The listing builds one solid part. Answer for the finished solid, in the listing's coordinates (mm). Face numbers are marked on the shaded views. A direction names the side the tool comes from. Coordinates: 2 decimals unless noted, no trailing zeros. Write each loop counter-clockwise with the first axis right and the second up, starting at its lowest first coordinate (ties: lowest second). Pieces come first, ordered by that corner, then holes.
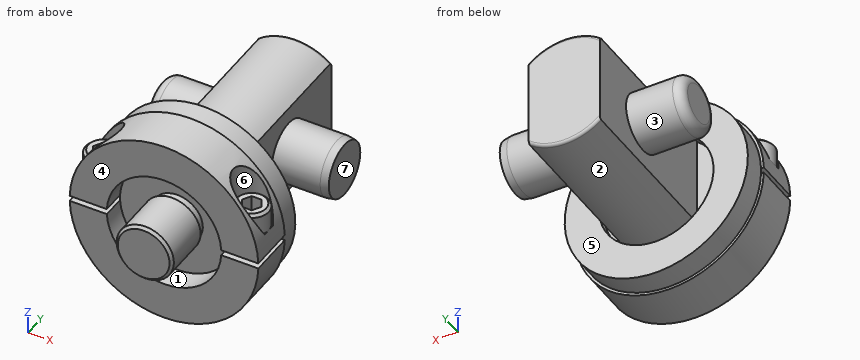
from build123d import *

# Parameters (mm, degrees)
FILLET1_R                  = 0.7874
SKETCH2_W                  = 6.0198
SKETCH2_H                  = 46.736
CUT_EXTRUDE1_DEPTH         = 16.875
CUT_EXTRUDE1_DEPTH_BACK    = 16.875
SKETCH3_R                  = 7.9375
SKETCH3_R_2                = 7.0866
CUT_EXTRUDE2_DEPTH         = 2.54
CHAMFER1_SIZE              = 0.762
SKETCH4_R                  = 7.94004
EXTRUDE1_DEPTH             = 25.4
CHAMFER2_SIZE              = 0.381
CHAMFER2_SIZE2             = 2.160758373
FILLET2_R                  = 2.6416
EXTRUDE2_DEPTH             = 6.35
EXTRUDE2_DEPTH_BACK        = 6.35
CUT_EXTRUDE3_START         = 5.588
SKETCH6_R                  = 5.1562
CUT_EXTRUDE3_DEPTH         = 20.812
SKETCH7_R                  = 4.7625
EXTRUDE3_DEPTH             = 6.35
CHAMFER3_SIZE              = 0.762
CUT_EXTRUDE4_DEPTH         = 4.7625
EXTRUDE4_REACH             = 28.162
SKETCH10_R                 = 3.175
EXTRUDE4_DIRECTION_2_REACH = 28.162
SKETCH11_R                 = 25.4
SKETCH11_R_2               = 15.875
EXTRUDE5_DEPTH             = 6.35


with BuildPart() as part:
    # Sketch1 → Revolve1 (revolve)
    with BuildSketch(Plane(origin=(0, 0, 0), x_dir=(0, 0, -1), z_dir=(1, 0, 0))):
        Polygon((0, 56.896), (15.875, 56.896), (15.875, 0), (7.9375, 0), (7.9375, -16.129), (0, -16.129), align=None)
    revolve(axis=Axis((0, -15.35938, 0), (0, 1, 0)))

    # Fillet1
    fillet1_edges = [part.edges().sort_by_distance(p)[0] for p in [
        (0, 56.896, 15.875),
    ]]
    fillet(fillet1_edges, radius=FILLET1_R)

    # Sketch2 → Cut-Extrude1 (cut, two sides)
    with BuildSketch(Plane.XY) as cut_extrude1_sk:
        with Locations((12.8651, 33.528)):
            Rectangle(SKETCH2_W, SKETCH2_H)
        with Locations((-12.8651, 33.528)):
            Rectangle(SKETCH2_W, SKETCH2_H)
    extrude(amount=CUT_EXTRUDE1_DEPTH, mode=Mode.SUBTRACT)
    extrude(cut_extrude1_sk.sketch, amount=-CUT_EXTRUDE1_DEPTH_BACK, mode=Mode.SUBTRACT)

    # Sketch3 → Cut-Extrude2 (cut)
    with BuildSketch(Plane.XZ):
        with Locations(Location((0, 0, 0), (0, 0, 270))):  # turned: the seam where the file's is
            Circle(SKETCH3_R)
        with Locations(Location((0, 0, 0), (0, 0, 270))):  # turned: the seam where the file's is
            Circle(SKETCH3_R_2, mode=Mode.SUBTRACT)
    extrude(amount=CUT_EXTRUDE2_DEPTH, mode=Mode.SUBTRACT)

    # Chamfer1
    chamfer1_edges = [part.edges().sort_by_distance(p)[0] for p in [
        (0, -16.129, 7.9375),
    ]]
    chamfer(chamfer1_edges, length=CHAMFER1_SIZE)

    # Sketch4 → Extrude1 (add, symmetric)
    with BuildSketch(Plane(origin=(0, 0, 0), x_dir=(0, 0, -1), z_dir=(1, 0, 0))):
        with Locations(Location((0, 36.322, 0), (0, 0, 90))):  # turned: the seam where the file's is
            Circle(SKETCH4_R)
    extrude(amount=EXTRUDE1_DEPTH, both=True)

    # Chamfer2
    chamfer2_edges = [part.edges().sort_by_distance(p)[0] for p in [
        (25.4, 28.38196, 0),
    ]]
    chamfer2_side = [part.faces().sort_by_distance(p)[0] for p in [
        (25.4, 36.322, 0),
    ]]
    chamfer(chamfer2_edges, length=CHAMFER2_SIZE, length2=CHAMFER2_SIZE2, reference=chamfer2_side[0])

    # Fillet2
    fillet2_edges = [part.edges().sort_by_distance(p)[0] for p in [
        (-25.4, 28.38196, 0),
    ]]
    fillet(fillet2_edges, radius=FILLET2_R)

    # Sketch5 → Extrude2 (add, two sides)
    with BuildSketch(Plane(origin=(0, 0, 0), x_dir=(1, 0, 0), z_dir=(0, 1, 0))) as extrude2_sk:
        with BuildLine():
            Line((15.856701454, 0.762), (26.150900558, 0.762))
            ThreePointArc((26.150900558, 0.762), (0, 26.162), (-26.150900558, 0.762))
            Line((-26.150900558, 0.762), (-15.856701454, 0.762))
            ThreePointArc((-15.856701454, 0.762), (0, 15.875), (15.856701454, 0.762))
        make_face()
        with BuildLine():
            Line((15.856701454, -0.762), (26.150900558, -0.762))
            ThreePointArc((26.150900558, -0.762), (0, -26.162), (-26.150900558, -0.762))
            Line((-26.150900558, -0.762), (-15.856701454, -0.762))
            ThreePointArc((-15.856701454, -0.762), (0, -15.875), (15.856701454, -0.762))
        make_face()
    extrude(amount=EXTRUDE2_DEPTH)
    extrude(extrude2_sk.sketch, amount=-EXTRUDE2_DEPTH_BACK)

    # Sketch6 → Cut-Extrude3 (cut, through all)
    with BuildSketch(Plane.XY.offset(0.762).offset(CUT_EXTRUDE3_START)):
        with Locations((20.6375, 0)):
            Circle(SKETCH6_R)
        with Locations((-20.6375, 0)):
            Circle(SKETCH6_R)
    extrude(amount=CUT_EXTRUDE3_DEPTH, mode=Mode.SUBTRACT)

    # Sketch7 → Extrude3 (add)
    with BuildSketch(Plane.XY.offset(6.35)):
        with Locations(Location((20.6375, 0, 0), (0, 0, 5.295701499))):  # turned: the seam where the file's is
            Circle(SKETCH7_R)
        with Locations(Location((-20.6375, 0, 0), (0, 0, 185.295701499))):  # turned: the seam where the file's is
            Circle(SKETCH7_R)
    extrude(amount=EXTRUDE3_DEPTH)

    # Chamfer3
    chamfer3_edges = [part.edges().sort_by_distance(p)[0] for p in [
        (15.895328135, -0.439559152, 12.7),
        (-15.895328135, 0.439559152, 12.7),
    ]]
    chamfer(chamfer3_edges, length=CHAMFER3_SIZE)

    # Sketch8 → Cut-Extrude4 (cut)
    with BuildSketch(Plane.XY.offset(12.7)):
        Polygon((22.012315329, 2.38125), (23.387130657, 0), (22.012315329, -2.38125), (19.262684671, -2.38125), (17.887869343, 0), (19.262684671, 2.38125), align=None)
        Polygon((-23.387130657, 0), (-22.012315329, -2.38125), (-19.262684671, -2.38125), (-17.887869343, 0), (-19.262684671, 2.38125), (-22.012315329, 2.38125), align=None)
    extrude(amount=-CUT_EXTRUDE4_DEPTH, mode=Mode.SUBTRACT)

    # Sketch10 → Extrude4 (add, up to next)
    with BuildSketch(Plane.XY, mode=Mode.PRIVATE) as extrude4_sk1:
        with Locations((20.6375, 0)):
            Circle(SKETCH10_R)
    extrude4_tool1 = extrude(extrude4_sk1.sketch, amount=EXTRUDE4_REACH, mode=Mode.PRIVATE) - part.part
    add(extrude4_tool1.solids().sort_by_distance((20.6375, 0, 0))[0])
    # Sketch10 → Extrude4 (add, up to next)
    with BuildSketch(Plane.XY, mode=Mode.PRIVATE) as extrude4_sk2:
        with Locations((-20.6375, 0)):
            Circle(SKETCH10_R)
    extrude4_tool2 = extrude(extrude4_sk2.sketch, amount=EXTRUDE4_REACH, mode=Mode.PRIVATE) - part.part
    add(extrude4_tool2.solids().sort_by_distance((-20.6375, 0, 0))[0])

    # Sketch10 → Extrude4 direction 2 (add, up to next)
    with BuildSketch(Plane.XY, mode=Mode.PRIVATE) as extrude4_direction_2_sk1:
        with Locations((20.6375, 0)):
            Circle(SKETCH10_R)
    extrude4_direction_2_tool1 = extrude(extrude4_direction_2_sk1.sketch, amount=-EXTRUDE4_DIRECTION_2_REACH, mode=Mode.PRIVATE) - part.part
    add(extrude4_direction_2_tool1.solids().sort_by_distance((20.6375, 0, 0))[0])
    # Sketch10 → Extrude4 direction 2 (add, up to next)
    with BuildSketch(Plane.XY, mode=Mode.PRIVATE) as extrude4_direction_2_sk2:
        with Locations((-20.6375, 0)):
            Circle(SKETCH10_R)
    extrude4_direction_2_tool2 = extrude(extrude4_direction_2_sk2.sketch, amount=-EXTRUDE4_DIRECTION_2_REACH, mode=Mode.PRIVATE) - part.part
    add(extrude4_direction_2_tool2.solids().sort_by_distance((-20.6375, 0, 0))[0])

    # Sketch11 → Extrude5 (add)
    with BuildSketch(Plane(origin=(0, 6.35, 0), x_dir=(-1, 0, 0), z_dir=(0, 1, 0))):
        with Locations(Location((0, 0, 0), (0, 0, 181.719131321))):  # turned: the seam where the file's is
            Circle(SKETCH11_R)
        Circle(SKETCH11_R_2, mode=Mode.SUBTRACT)
    extrude(amount=EXTRUDE5_DEPTH)


solid = part.part
1. Section C-C on z = 19.5 is taken. Give the vertices of the cut face in (x, y), then the cut area to 3 significant figures.
Results found:
outline: (-17.44, -6.35) - (17.44, -6.35) - (17.44, -4.05) arc R5.16 cw to (17.44, 4.05) - (17.44, 6.35) - (16.28, 6.35) - (16.28, 12.7) - (-16.28, 12.7) - (-16.28, 6.35) - (-17.44, 6.35) - (-17.44, 4.05) arc R5.16 cw to (-17.44, -4.05) - close
area: 628 mm2
2. Flat-ended cylindrical pins translate along their axes: P1, Ø5, axis at x = 19, y = -1, coming from the -Z side; P2, Ø6.5, axis at x = 22, y = 0, coming from the +Z side; P3, Ø12, axis at x = 9.5, y = 31, coming from the -Z side; P4, Ø4, axis at x = -19, y = 48, coming from the +Z side. Find the tip coordinate at first contact, or state that the pin passes through.
Results found:
P1: stops at z = -20.3
P2: stops at z = 12.7
P3: stops at z = -15.48
P4: passes through
3. Find the intervals of material crossed by L1, parallel to Z at x = -4.5, y = -5; L2, parallel to Z at x = -3.5, y = -4; L3, parallel to Y at x = 10.5, z = -19.5, in increasing order.
Results found:
L1: z = -25.77 to -15.22, -6.54 to 6.54, 15.22 to 25.77
L2: z = -25.93 to -15.48, -7.12 to 7.12, 15.48 to 25.93
L3: y = -6.35 to 12.7
4. A tool of negligible diameter and unlimited length cuts with its end or side. For the marked faces 4, 5, 6 and 7, from which of +Z, -Z, +X, -X, +Y, -Y can it reach the whole face along a straight path? Write none if from no direction.
Results found:
face 4: +Z, -Y
face 5: none
face 6: +Z
face 7: +Z, -Z, +X, +Y
5. Section D-D on y = -10.5 is taken. Give the vertices of the cut face in (x, z) (1 decimal).
Results found:
outline: circle Ø15.9 at (0, 0)
6. Section B-B on z = 9 is taken. State how many separate pieces and enclosed holes the cut face has, then the cut area to 3 significant figures.
Results found:
separate pieces: 3
enclosed holes: 2
area: 1,560 mm2
7. For a pull along X with two mould halves and no side action, classify the marked faces 1, 2 and 3 as pulls with the +X half, pulls with the -X half, needs draft (parallel to the pull), parting line crosses it, or undercut.
Results found:
face 1: undercut
face 2: parting line crosses it
face 3: needs draft
